Design review of the part built by this model. Coordinates are the model's own, in mm. Face numbers are marked on the shaded views. A direction names the side the tool comes from. Round coordinates to 2 decimals unless told otherwise and drop trailing zeros. Order: outer loops, then holes, each group sorted by start corner. A loop starts at its lowest first (then second) coordinate and runs counter-clockwise, first axis right, second up.
from build123d import *

# Parameters (mm, degrees)
BOSS_EXTRUDE1_DEPTH     = 7.5
CUT_EXTRUDE1_DEPTH      = 37.827299657
CUT_EXTRUDE1_DEPTH_BACK = 37.827299657
SKETCH3_R               = 4.7625
FILLET1_R               = 7.5
SKETCH4_R               = 2.8067
CUT_EXTRUDE2_DEPTH      = 37.827299657


with BuildPart() as part:
    # Sketch1 → Boss-Extrude1 (new, symmetric)
    with BuildSketch(Plane(origin=(0, 0, 0), x_dir=(1, 0, 0), z_dir=(0, 1, 0))):
        Polygon((-15, -7.5), (-20, -7.5), (-20, 22.049394585), (-6.22914747, 30), (6.22914747, 30), (20, 22.049394585), (20, -7.5), (15, -7.5), (15, 19.226497308), (5, 25), (-5, 25), (-15, 19.226497308), align=None)
    extrude(amount=BOSS_EXTRUDE1_DEPTH, both=True)

    # Sketch3 → Cut-Extrude1 (cut, two sides: drawn at the far end of the back side and taken through both)
    with BuildSketch(Plane(origin=(0, 0, 0), x_dir=(0, 0, -1), z_dir=(1, 0, 0)).offset(-CUT_EXTRUDE1_DEPTH_BACK)):
        Circle(SKETCH3_R)
    extrude(amount=CUT_EXTRUDE1_DEPTH + CUT_EXTRUDE1_DEPTH_BACK, mode=Mode.SUBTRACT)

    # Fillet1
    fillet1_edges = [part.edges().sort_by_distance(p)[0] for p in [
        (17.5, 7.5, 7.5),
        (17.5, -7.5, 7.5),
        (-17.5, -7.5, 7.5),
        (-17.5, 7.5, 7.5),
    ]]
    fillet(fillet1_edges, radius=FILLET1_R - 0.0001)  # a hair under: the kernel refuses the full size

    # Sketch4 → Cut-Extrude2 (cut, through all)
    with BuildSketch(Plane.XY):
        Circle(SKETCH4_R)
    extrude(amount=-CUT_EXTRUDE2_DEPTH, mode=Mode.SUBTRACT)


solid = part.part
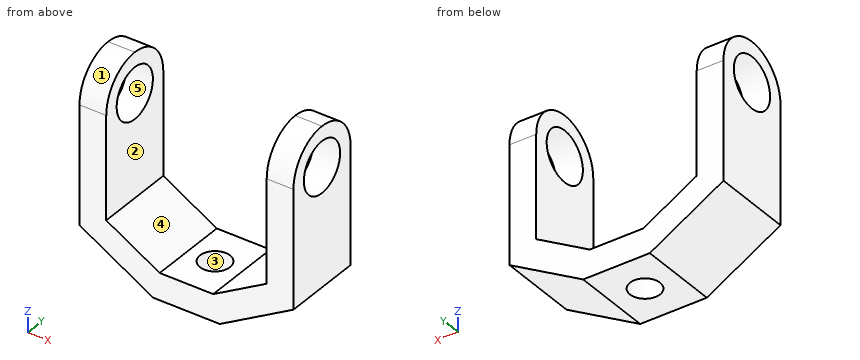
1) Clearance check with flat-ended pins moving along their axes: P1, Ø5, axis at x = -0.5, y = -1, coming from the +Z side; P2, Ø2, axis at x = 10, y = -3, coming from the -Z side; P3, Ø2, axis at x = -10.5, y = 4.5, coming from the +Z side. State where each tip first meets the part, or that it passes through.
Results:
P1: stops at z = -25
P2: stops at z = -28.4
P3: stops at z = -21.25
2) Take a section at B-B on x = 0. Give the boundary of the cut face in (y, z).
Results:
outline: (-7.5, -30) - (-2.81, -30) - (-2.81, -25) - (-7.5, -25) - close; (2.81, -30) - (7.5, -30) - (7.5, -25) - (2.81, -25) - close
3) Take a section at D-D on y = -0.75. Give the boundary of the cut face in (x, z), plus the area to 3 significant figures.
Results:
outline: (-20, -22.05) - (-6.23, -30) - (-2.7, -30) - (-2.7, -25) - (-5, -25) - (-15, -19.23) - (-15, -4.7) - (-20, -4.7) - close; (-20, 4.7) - (-15, 4.7) - (-15, 7.46) - (-20, 7.46) - close; (2.7, -30) - (6.23, -30) - (20, -22.05) - (20, -4.7) - (15, -4.7) - (15, -19.23) - (5, -25) - (2.7, -25) - close; (15, 4.7) - (20, 4.7) - (20, 7.46) - (15, 7.46) - close
area: 352 mm2
4) Take a section at A-A on z = -13. Give the boundary of the cut face in (x, y), plus the area to 3 significant figures.
Results:
outline: (-20, -7.5) - (-15, -7.5) - (-15, 7.5) - (-20, 7.5) - close; (15, -7.5) - (20, -7.5) - (20, 7.5) - (15, 7.5) - close
area: 150 mm2
5) The part is to be moulded in two halves that separate along Y. For the marked faces 1, 2 and 3, say which applies: released by +Y, released by -Y, zero draft, split by the parting line, or undercut.
Results:
face 1: released by -Y
face 2: zero draft
face 3: undercut
6) To check wall thickness, follow line 1 along X through (y, z) = (0, 6); line 2 along Y through (x, z) = (0, -26); line 3 along Y through (x, z) = (-18, 0). State the ranges of each line that lie inside material, in increasing order.
Results:
line 1: x = -20 to -15, 15 to 20
line 2: y = -7.5 to -2.81, 2.81 to 7.5
line 3: y = -7.5 to -4.76, 4.76 to 7.5
7) Take a section at C-C on z = -0.5. Give the boundary of the cut face in (x, y).
Results:
outline: (-20, -7.5) - (-15, -7.5) - (-15, -4.74) - (-20, -4.74) - close; (-20, 4.74) - (-15, 4.74) - (-15, 7.5) - (-20, 7.5) - close; (15, -7.5) - (20, -7.5) - (20, -4.74) - (15, -4.74) - close; (15, 4.74) - (20, 4.74) - (20, 7.5) - (15, 7.5) - close
8) For the marked faces 4 and 5, list the 3-axis set-ups (+Z, -Z, +X, -X, +Y, -Y) from which the entire face can be reached by the end or side of a thin tool; tool diameter is ignored.
Results:
face 4: +Z, +Y, -Y
face 5: +X, -X
